Autodesk Inventor part; units mm, degrees
ref_plane "YZ Plane" through (0, 0, 0) normal (1, 0, 0) x (0, 1, 0)
ref_plane "XZ Plane" through (0, 0, 0) normal (0, 1, 0) x (-1, 0, 0)
ref_plane "XY Plane" through (0, 0, 0) normal (0, 0, 1) x (1, 0, 0)
sketch "Boceto3" plane through (0, 0, 0) normal (1, 0, 0) x (0, 1, 0)
  line L0 (0, 0) -> (0, -9)
  line L1 (0, -9) -> (13, -9)
  line L2 (13, -9) -> (13, 0)
  line L3 (13, 0) -> (0, 0)
  circle A0 centre (6.5, -4.5) radius 0.9
  dimension "d3" = 9
  dimension "d4" = 13
  dimension "d7" = 1.8
extrude "Extrusión1" add sketch "Boceto3" along normal blind 10.06
sketch "Boceto4" plane through (10.06, 0, 0) normal (1, 0, 0) x (0, 0, -1)
  point P0 (0, 0)
  point P1 (4.4995, 6.4877)
hole "Agujero1" at (10.06, 6.4877, -4.4995) direction (-1, 0, 0) diameter 4 depth 9
fillet "Empalme1" radius 1 4 edges at (5.03, 13, 0) (5.03, 13, -9) (5.03, 0, 0) (5.03, 0, -9)
properties part number "Soporte placa B1 - B2"
Work out the finished part from the listing and answer in its coordinate system (mm). A direction names the side the tool comes from. Give positions to 0.01 mm unless a question says otherwise; leave off trailing zeros. Order: outer loops, then holes, each group sorted by start corner. A loop starts at its lowest first (then second) coordinate and runs counter-clockwise, first axis right, second up. Notation, with made-up numbers: (-24, 21) - (3, 21) arc R7 cw to (3, 28) - close; hole circle Ø3 at (82, 66). An arc over 180 degrees is marked (long way). One line per item, written item: value. Start each with the question number.
1. Consider line 1 (Z direction, x = 0.35, y = 6.5); line 2 (Y direction, x = 0.4, z = -4.5); line 3 (Y direction, x = 7, z = -4.5). Determine where each line is inside the solid, lowest interval first.
2. For a pull along Y with two mould halves and no side action, classify faces 3 (the face through (0.523, 6.305, -3.621)), 4 (the face through (10.06, 6, -2)), 5 (the face through (5, 0, -4)) as released by +Y, released by -Y, zero draft, split by the parting line, or undercut.
3. Section A-A, the plane z = -4.5 is taken. Write down the section's boundary in (x, y).
4. Section B-B, the plane x = 7.5 is taken. Write down the section's boundary in (y, z), then the cut area to 3 significant figures.
5. Which of the six approach directions +Z, -Z, +X, -X, +Y, -Y give full straight-line access (tool end or side, diameter ignored) to faces 1 (the face through (5, 13, -5)), 2 (the face through (5.5, 5.89, -6.41))?
Filled sheet:
1. line 1: -9 to -5.4, -3.6 to 0
1. line 2: 0 to 5.6, 7.4 to 13
1. line 3: 0 to 4.49, 8.49 to 13
2. face 3: undercut
2. face 4: zero draft
2. face 5: released by -Y
3. outline: (0, 0) - (10.06, 0) - (10.06, 4.49) - (1.06, 4.49) - (1.06, 5.6) - (0, 5.6) - close; (0, 7.4) - (1.06, 7.4) - (1.06, 8.49) - (10.06, 8.49) - (10.06, 13) - (0, 13) - close
4. outline: (0, -8) arc R1 ccw to (1, -9) - (12, -9) arc R1 ccw to (13, -8) - (13, -1) arc R1 ccw to (12, 0) - (1, 0) arc R1 ccw to (0, -1) - close; hole circle Ø4 at (6.49, -4.5)
4. area: 104 mm²
5. face 1: +Z, -Z, +X, -X, +Y
5. face 2: +X
